Design review of the part built by this model. Coordinates are the model's own, in mm. A direction names the side the tool comes from. Round coordinates to 2 decimals unless told otherwise and drop trailing zeros. Loops run counter-clockwise (first coordinate to the right, second up) from the corner with the lowest first, then second, coordinate; pieces in that order, holes last. Notation, with made-up numbers: M 46,-33 L 105,-33 A22 cw 105,-24 Z; hole C -39,61.25 d2. An arc over 180 degrees is marked long. One line per item, written item: value. Start each with the question number.
Item 1: We need section C-C (y = 0). Write out the cut boundary in (x, z), then the cut area to 3 significant figures.
Item 2: We need section B-B (x = -13.1). Write out the cut boundary in (y, z).
Item 3: We need section A-A (z = 1.05). Write out the cut boundary in (x, y).
Item 4: We need section D-D (x = 0). Write out the cut boundary in (y, z), then the cut area to 3 significant figures.
Item 5: Mouldability with a two-part tool opening along Y and no side actions: class faces 1 (the flat face through (-25, 0, 1)), 2 (the cylindrical face through (-24.43, -4.65, 1.01)), 3 (the cylindrical face through (-14.85, 0.08, 0.99)) as released by +Y, released by -Y, zero draft, split by the parting line, or undercut.
Item 6: For faces 4 (the flat face through (9.5, 0, 1)), 5 (the cylindrical face through (24.4, -4.68, 1.01)), list the 3-axis set-ups (+Z, -Z, +X, -X, +Y, -Y) from which the entire face can be reached by the end or side of a thin tool; tool diameter is ignored.
Item 7: For line 1 along X through (y, z) = (2.25, 1.8); line 2 along Y through (x, z) = (-13.1, 1.35); line 3 along X through (y, z) = (0.75, 1.6), list the stretches that pass through material, from the lowest coordinate up.
from build123d import *

# Parameters (mm, degrees)
SKETCH_1_W          = 50
SKETCH_1_H          = 10.5
SKETCH_1_R          = 1.75
EXTRUDE_1_DEPTH     = 2
FILLET_1_R          = 2
SKETCH_2_W          = 19
SKETCH_2_H          = 10.5
CUT_EXTRUDE_1_DEPTH = 1.8
SKETCH_3_R          = 3
CUT_EXTRUDE_2_DEPTH = 3


with BuildPart() as part:
    # ｽｹｯﾁ1 → ﾎﾞｽ - 押し出し1 (new body)
    with BuildSketch(Plane.XY):
        Rectangle(SKETCH_1_W, SKETCH_1_H)
        with Locations((13.1, 0)):
            Circle(SKETCH_1_R, mode=Mode.SUBTRACT)
        with Locations((-13.1, 0)):
            Circle(SKETCH_1_R, mode=Mode.SUBTRACT)
    extrude(amount=EXTRUDE_1_DEPTH)

    # ﾌｨﾚｯﾄ1
    fillet_1_edges = [part.edges().sort_by_distance(p)[0] for p in [
        (25, -5.25, 1),
        (-25, -5.25, 1),
        (-25, 5.25, 1),
        (25, 5.25, 1),
    ]]
    fillet(fillet_1_edges, radius=FILLET_1_R)

    # ｽｹｯﾁ2 → ｶｯﾄ - 押し出し1 (cut)
    with BuildSketch(Plane.XY.offset(2)):
        Rectangle(SKETCH_2_W, SKETCH_2_H)
    extrude(amount=-CUT_EXTRUDE_1_DEPTH, mode=Mode.SUBTRACT)

    # ｽｹｯﾁ3 → ｶｯﾄ - 押し出し2 (cut, through all)
    with BuildSketch(Plane(origin=(0, 0, 0), x_dir=(-1, 0, 0), z_dir=(0, 0, -1))):
        Circle(SKETCH_3_R)
    extrude(amount=-CUT_EXTRUDE_2_DEPTH, mode=Mode.SUBTRACT)


solid = part.part
A:
1. outline: M -25,0 L -14.85,0 L -14.85,2 L -25,2 Z; M -11.35,0 L -3,0 L -3,0.2 L -9.5,0.2 L -9.5,2 L -11.35,2 Z; M 3,0 L 11.35,0 L 11.35,2 L 9.5,2 L 9.5,0.2 L 3,0.2 Z; M 14.85,0 L 25,0 L 25,2 L 14.85,2 Z
1. area: 50.6 mm2
2. outline: M -5.25,0 L -1.75,0 L -1.75,2 L -5.25,2 Z; M 1.75,0 L 5.25,0 L 5.25,2 L 1.75,2 Z
3. outline: M -25,-3.25 A2 ccw -23,-5.25 L -9.5,-5.25 L -9.5,5.25 L -23,5.25 A2 ccw -25,3.25 Z; M 9.5,-5.25 L 23,-5.25 A2 ccw 25,-3.25 L 25,3.25 A2 ccw 23,5.25 L 9.5,5.25 Z; hole C -13.1,0 d3.5; hole C 13.1,0 d3.5
4. outline: M -5.25,0 L -3,0 L -3,0.2 L -5.25,0.2 Z; M 3,0 L 5.25,0 L 5.25,0.2 L 3,0.2 Z
4. area: 0.900 mm2
5. face 1: zero draft
5. face 2: released by -Y
5. face 3: undercut
6. face 4: +Z, +Y, -Y
6. face 5: +Z, -Z, +X, -Y
7. line 1: -25 to -9.5, 9.5 to 25
7. line 2: -5.25 to -1.75, 1.75 to 5.25
7. line 3: -25 to -14.68, -11.52 to -9.5, 9.5 to 11.52, 14.68 to 25
